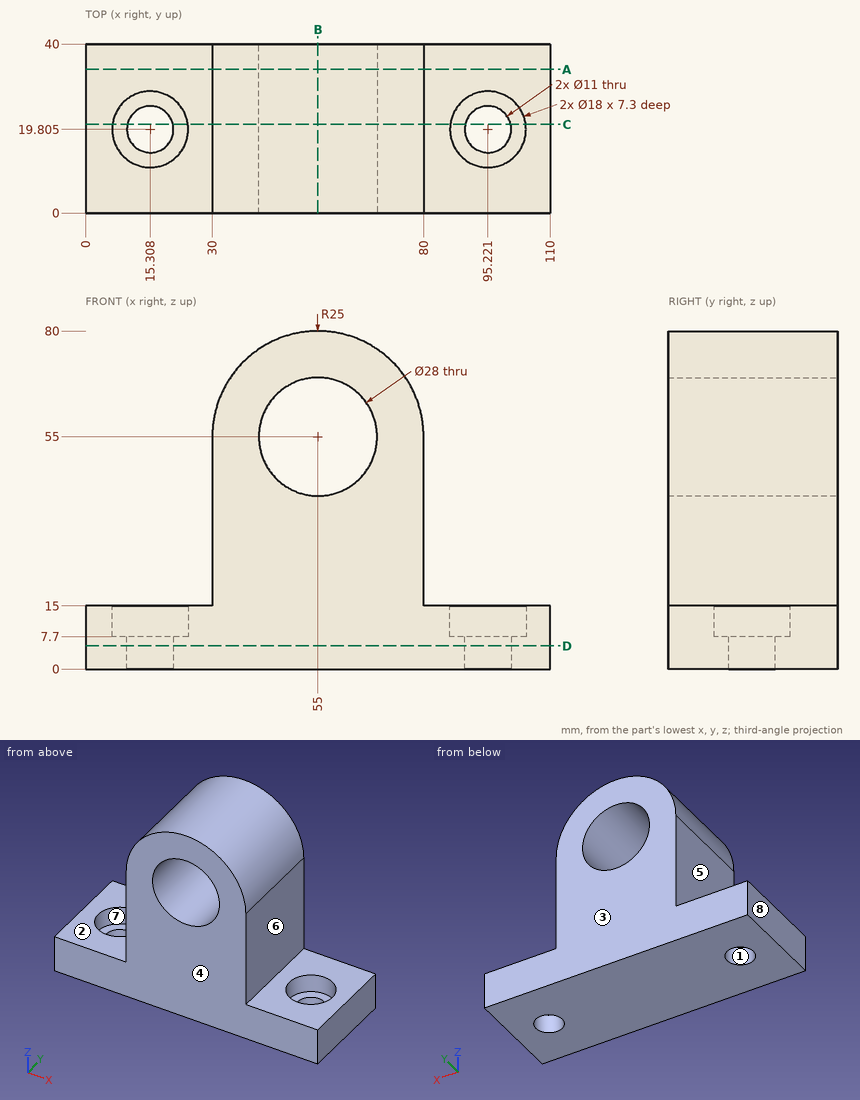
For this review, use the dimensioned drawing (mm, ordinates from the lowest corner) and the shaded views. A direction names the side the tool comes from. Coordinates: 2 decimals unless noted, no trailing zeros. Loops run counter-clockwise (first coordinate to the right, second up) from the corner with the lowest first, then second, coordinate; pieces in that order, holes last. Notation, with made-up numbers: (6.25, -17) -> (14.25, -17) arc R19 cw to (14.25, 12) -> close; hole circle Ø8 at (11, 16.5). An arc over 180 degrees is marked (long way). Use a Markdown table: item, result. Add a question column.
Item 1: Clearance check with flat-ended pins moving along their axes: P1, Ø2, axis at x = 31.5, y = 16.5, coming from the +Z side (1 decimal); P2, Ø6, axis at x = 18.5, y = 24.5, coming from the +Z side; P3, Ø8, axis at x = 46, z = 51, coming from the -Y side; P4, Ø2, axis at x = 54, y = 5, coming from the +Z side. State where each tip first meets the part, or that it passes through.
Item 2: We need section C-C, the plane y = 21. Write out the cut boundary in (x, z), and give its area (3 significant figures).
Item 3: We need section D-D, the plane z = 5.5. Write out the cut boundary in (x, y) (1 decimal).
Item 4: Wall thickness on L1, parallel to Z at x = 55, y = 12; L2, parallel to Z at x = 101, y = 38.5; L3, parallel to X at y = 28, z = 51.5 (1 decimal): over which ranges is each line inside the solid? List them lowest first. Write a range as from..to.
Item 5: The part is to be moulded in two halves that separate along Y. For the marked faces 1, 2, 3 and 4, say which applies: +Y half, -Y half, draft (parallel to the pull), parting line (faces both ways), or undercut.
Item 6: We need section A-A, the plane y = 34. Write out the cut boundary in (x, z).
Item 7: We need section B-B, the plane x = 55. Write out the cut boundary in (y, z), and give its area (3 significant figures).
Item 8: Machinability: for the marked faces 5, 6, 7 and 8, which of the approach directions +Z, -Z, +X, -X, +Y, -Y give a long, thin tool a straight path to every point of the face, cutting with its end or side? Answer none if there is none.
Numbers:
| question | item | result |
|---|---|---|
| 1 | P1 | stops at z = 65.9 |
| 1 | P2 | stops at z = 7.7 |
| 1 | P3 | passes through |
| 1 | P4 | stops at z = 80 |
| 2 | outline | (0, 0) -> (9.94, 0) -> (9.94, 7.7) -> (6.39, 7.7) -> (6.39, 15) -> (0, 15) -> close; (20.68, 0) -> (89.85, 0) -> (89.85, 7.7) -> (86.3, 7.7) -> (86.3, 15) -> (80, 15) -> (80, 55) arc R25 ccw to (30, 55) -> (30, 15) -> (24.23, 15) -> (24.23, 7.7) -> (20.68, 7.7) -> close; (100.59, 0) -> (110, 0) -> (110, 15) -> (104.14, 15) -> (104.14, 7.7) -> (100.59, 7.7) -> close; hole circle Ø28 at (55, 55) |
| 2 | area | 3,590 mm^2 |
| 3 | outline | (0, 0) -> (110, 0) -> (110, 40) -> (0, 40) -> close; hole circle Ø11 at (15.3, 19.8); hole circle Ø11 at (95.2, 19.8) |
| 4 | L1 | z = 0..41, 69..80 |
| 4 | L2 | z = 0..15 |
| 4 | L3 | x = 30..41.4, 68.6..80 |
| 5 | face 1 | undercut |
| 5 | face 2 | draft |
| 5 | face 3 | +Y half |
| 5 | face 4 | -Y half |
| 6 | outline | (0, 0) -> (110, 0) -> (110, 15) -> (80, 15) -> (80, 55) arc R25 ccw to (30, 55) -> (30, 15) -> (0, 15) -> close; hole circle Ø28 at (55, 55) |
| 7 | outline | (0, 0) -> (40, 0) -> (40, 41) -> (0, 41) -> close; (0, 69) -> (40, 69) -> (40, 80) -> (0, 80) -> close |
| 7 | area | 2,080 mm^2 |
| 8 | face 5 | +Z, -X, +Y, -Y |
| 8 | face 6 | +Z, +X, +Y, -Y |
| 8 | face 7 | +Z |
| 8 | face 8 | +Z, -Z, -X, +Y, -Y |
